CAD build for the part. Positions are in the model's coordinates, mm. Face numbers are marked on the shaded views. Round coordinates to 2 decimals unless told otherwise and drop trailing zeros. Order: outer loops, then holes, each group sorted by start corner. A loop starts at its lowest first (then second) coordinate and runs counter-clockwise, first axis right, second up.
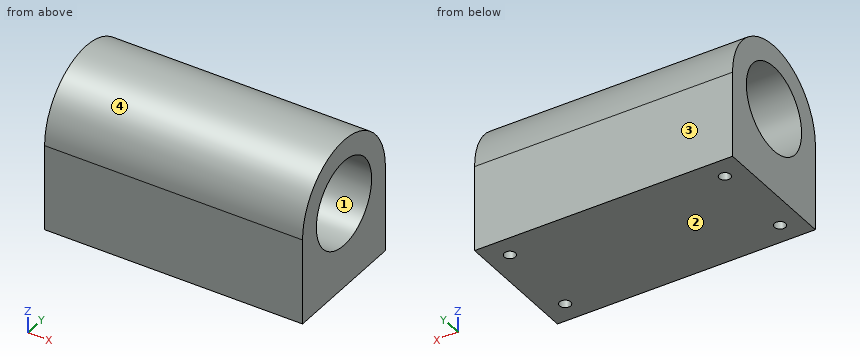
```python
from build123d import *

# Parameters (mm, degrees)
F1_DEPTH = 30
F2_R     = 0.65
F3_DEPTH = 5


with BuildPart() as f1:
    # F0 (on Right) → F1 (new body)
    with BuildSketch(Plane.YZ):
        with BuildLine():
            ThreePointArc((-5, 0), (0, 5), (5, 0))
            Line((5, 0), (7.5, 0))
            ThreePointArc((7.5, 0), (0, 7.5), (-7.5, 0))
            Line((-7.5, 0), (-5, 0))
        make_face()
        with BuildLine():
            Line((7.5, 0), (5, 0))
            ThreePointArc((5, 0), (0, -5), (-5, 0))
            Line((-5, 0), (-7.5, 0))
            Line((-7.5, 0), (-7.5, -10))
            Line((-7.5, -10), (7.5, -10))
            Line((7.5, -10), (7.5, 0))
        make_face()
    extrude(amount=F1_DEPTH)

    # F2 (on face) → F3 (cut)
    with BuildSketch(Plane(origin=(0, 0, -10), x_dir=(1, 0, 0), z_dir=(0, 0, -1))):
        with Locations((27.5, 5)):
            Circle(F2_R)
        with Locations((27.5, -5)):
            Circle(F2_R)
        with Locations((2.5, 5)):
            Circle(F2_R)
        with Locations((2.5, -5)):
            Circle(F2_R)
    extrude(amount=-F3_DEPTH, mode=Mode.SUBTRACT)


solid = f1.part
```
1. Cut at B-B, the plane y = 0. Write the cut outline in (x, z), and give its area (3 significant figures).
2. Mould opens along Z. For the marked faces 1, 2, 3 and 4 say: released by +Z, released by -Z, zero draft, split by the parting line, or undercut.
3. Drill centre lines: line 1 (Y direction, x = 27.5, z = -6.7); line 2 (Z direction, x = 9.75, y = -0.25); line 3 (Y direction, x = 27, z = -6.75). Where is each one in solid material? Low to high.
4. Cut at C-C, the plane z = -1. Write the cut outline in (x, y).
5. Cut at A-A, the plane x = 27.5. Write the cut outline in (y, z).
6. Cut at D-D, the plane x = 12.75. Write the cut outline in (y, z), and give its area (3 significant figures).
7. Pin check, flat tips, straight feed: P1, Ø1.5, axis at x = 14, y = -2.5, coming from the +Z side; P2, Ø1.7, axis at x = 2.5, y = 5, coming from the -Z side; P3, Ø1, axis at x = 27.5, y = 5, coming from the -Z side; P4, Ø2, axis at x = 2.5, y = -5, coming from the +Z side. Stop position of each tip, or through.
Outcome:
1. outline: (0, -10) - (30, -10) - (30, -5) - (0, -5) - close; (0, 5) - (30, 5) - (30, 7.5) - (0, 7.5) - close
1. area: 225 mm2
2. face 1: undercut
2. face 2: released by -Z
2. face 3: zero draft
2. face 4: released by +Z
3. line 1: y = -7.5 to -5.65, -4.35 to 4.35, 5.65 to 7.5
3. line 2: z = -10 to -4.99, 4.99 to 7.5
3. line 3: y = -7.5 to -5.42, -4.58 to 4.58, 5.42 to 7.5
4. outline: (0, -7.5) - (30, -7.5) - (30, -4.9) - (0, -4.9) - close; (0, 4.9) - (30, 4.9) - (30, 7.5) - (0, 7.5) - close
5. outline: (-7.5, -10) - (-5.65, -10) - (-5.65, -5) - (-4.35, -5) - (-4.35, -10) - (4.35, -10) - (4.35, -5) - (5.65, -5) - (5.65, -10) - (7.5, -10) - (7.5, 0) arc R7.5 ccw to (-7.5, 0) - close; hole circle Ø10 at (0, 0)
6. outline: (-7.5, -10) - (7.5, -10) - (7.5, 0) arc R7.5 ccw to (-7.5, 0) - close; hole circle Ø10 at (0, 0)
6. area: 160 mm2
7. P1: stops at z = 7.29
7. P2: stops at z = -10
7. P3: stops at z = -5
7. P4: stops at z = 6.34
